```python
from build123d import *

# Parameters (mm, degrees)
CROQUIS1_W              = 65
CROQUIS1_H              = 65
CROQUIS1_R              = 5.1
CROQUIS1_R_2            = 6
CROQUIS1_R_3            = 4.6
SALIENTE_EXTRUIR1_DEPTH = 5
REDONDEO2_R             = 3
CROQUIS2_R              = 4.6
SALIENTE_EXTRUIR2_DEPTH = 1
CROQUIS3_R              = 2.5
CORTAR_EXTRUIR1_DEPTH   = 1
CROQUIS4_R              = 2.4
CORTAR_EXTRUIR2_DEPTH   = 10
CROQUIS5_R              = 2.4
CROQUIS5_R_2            = 1.25
SALIENTE_EXTRUIR3_DEPTH = 2.4
SALIENTE_EXTRUIR4_START = -2
CROQUIS6_R              = 5.1
SALIENTE_EXTRUIR4_DEPTH = 2


with BuildPart() as part:
    # Croquis1 → Saliente-Extruir1 (new body)
    with BuildSketch(Plane.XZ):
        with Locations((-15.241230111, -32.770729042)):
            Rectangle(CROQUIS1_W, CROQUIS1_H)
        with Locations((-35.389174066, -12.520729042)):
            Circle(CROQUIS1_R, mode=Mode.SUBTRACT)
        with Locations((4.310825934, -12.520729042)):
            Circle(CROQUIS1_R, mode=Mode.SUBTRACT)
        with Locations((-35.389174066, -52.520729042)):
            Circle(CROQUIS1_R, mode=Mode.SUBTRACT)
        with Locations((4.310825934, -52.520729042)):
            Circle(CROQUIS1_R, mode=Mode.SUBTRACT)
        with Locations((4.310825934, -32.520729042)):
            Circle(CROQUIS1_R_2, mode=Mode.SUBTRACT)
        with Locations((-35.389174066, -32.520729042)):
            Circle(CROQUIS1_R_3, mode=Mode.SUBTRACT)
        with BuildLine():
            Line((-32.439174066, -6.320729042), (-38.939173538, -6.320729042))
            ThreePointArc((-38.939173538, -6.320729042), (-40.439173538, -4.820729042), (-38.939173538, -3.320729042))
            Line((-38.939173538, -3.320729042), (-32.439174066, -3.320729042))
            ThreePointArc((-32.439174066, -3.320729042), (-30.939174066, -4.820729042), (-32.439174066, -6.320729042))
        make_face(mode=Mode.SUBTRACT)
        with BuildLine():
            Line((7.860825934, -6.320729042), (1.360825562, -6.320729042))
            ThreePointArc((1.360825562, -6.320729042), (-0.139174438, -4.820729042), (1.360825562, -3.320729042))
            Line((1.360825562, -3.320729042), (7.860825934, -3.320729042))
            ThreePointArc((7.860825934, -3.320729042), (9.360825934, -4.820729042), (7.860825934, -6.320729042))
        make_face(mode=Mode.SUBTRACT)
        with BuildLine():
            Line((-38.939173538, -58.720729042), (-32.439174066, -58.720729042))
            ThreePointArc((-32.439174066, -58.720729042), (-30.939174066, -60.220729042), (-32.439174066, -61.720729042))
            Line((-32.439174066, -61.720729042), (-38.939173538, -61.720729042))
            ThreePointArc((-38.939173538, -61.720729042), (-40.439173538, -60.220729042), (-38.939173538, -58.720729042))
        make_face(mode=Mode.SUBTRACT)
        with BuildLine():
            Line((7.860825934, -61.720729042), (1.360825562, -61.720729042))
            ThreePointArc((1.360825562, -61.720729042), (-0.139174438, -60.220729042), (1.360825562, -58.720729042))
            Line((1.360825562, -58.720729042), (7.860825934, -58.720729042))
            ThreePointArc((7.860825934, -58.720729042), (9.360825934, -60.220729042), (7.860825934, -61.720729042))
        make_face(mode=Mode.SUBTRACT)
    extrude(amount=SALIENTE_EXTRUIR1_DEPTH)

    # Redondeo2
    redondeo2_edges = [part.edges().sort_by_distance(p)[0] for p in [
        (-47.741230111, -2.5, -0.270729042),
        (17.258769889, -2.5, -0.270729042),
        (17.258769889, -2.5, -65.270729042),
        (-47.741230111, -2.5, -65.270729042),
    ]]
    fillet(redondeo2_edges, radius=REDONDEO2_R)

    # Croquis2 → Saliente-Extruir2 (add)
    with BuildSketch(Plane(origin=(0, 0, 0), x_dir=(1, 0, 0), z_dir=(0, 1, 0))):
        with Locations(Location((-35.389174066, 32.520729042, 0), (0, 0, 180))):
            Circle(CROQUIS2_R)
    extrude(amount=-SALIENTE_EXTRUIR2_DEPTH)

    # Croquis3 → Cortar-Extruir1 (cut)
    with BuildSketch(Plane.XZ.offset(1)):
        with Locations((-35.389174066, -32.520729042)):
            Circle(CROQUIS3_R)
    extrude(amount=-CORTAR_EXTRUIR1_DEPTH, mode=Mode.SUBTRACT)

    # Croquis4 → Cortar-Extruir2 (cut)
    with BuildSketch(Plane.XZ.offset(5)):
        with Locations((-35.241230111, -44.020729042)):
            Circle(CROQUIS4_R)
        with Locations((-35.241230111, -21.520729042)):
            Circle(CROQUIS4_R)
        with Locations((4.758769889, -21.520729042)):
            Circle(CROQUIS4_R)
        with Locations((4.758769889, -44.020729042)):
            Circle(CROQUIS4_R)
    extrude(amount=-CORTAR_EXTRUIR2_DEPTH, mode=Mode.SUBTRACT)

    # Croquis5 → Saliente-Extruir3 (add)
    # profile 1 of 4: a face of its own
    with BuildSketch(Plane.XZ.offset(5)):
        with Locations((-35.241230111, -44.020729042)):
            Circle(CROQUIS5_R)
        with Locations((-35.241230111, -44.020729042)):
            Circle(CROQUIS5_R_2, mode=Mode.SUBTRACT)
    # profile 2 of 4: a face of its own
    with BuildSketch(Plane.XZ.offset(5)):
        with Locations((-35.241230111, -21.520729042)):
            Circle(CROQUIS5_R)
        with Locations((-35.241230111, -21.520729042)):
            Circle(CROQUIS5_R_2, mode=Mode.SUBTRACT)
    # profile 3 of 4: a face of its own
    with BuildSketch(Plane.XZ.offset(5)):
        with Locations((4.758769889, -21.520729042)):
            Circle(CROQUIS5_R)
        with Locations((4.758769889, -21.520729042)):
            Circle(CROQUIS5_R_2, mode=Mode.SUBTRACT)
    # profile 4 of 4: a face of its own
    with BuildSketch(Plane.XZ.offset(5)):
        with Locations((4.758769889, -44.020729042)):
            Circle(CROQUIS5_R)
        with Locations((4.758769889, -44.020729042)):
            Circle(CROQUIS5_R_2, mode=Mode.SUBTRACT)
    extrude(amount=-SALIENTE_EXTRUIR3_DEPTH)

    # Croquis6 → Saliente-Extruir4 (add)
    with BuildSketch(Plane.XZ.offset(5).offset(SALIENTE_EXTRUIR4_START)):
        with Locations((-35.389174066, -52.520729042)):
            Circle(CROQUIS6_R)
        with Locations((4.310825934, -52.520729042)):
            Circle(CROQUIS6_R)
        with Locations((4.310825934, -12.520729042)):
            Circle(CROQUIS6_R)
        with Locations((-35.389174066, -12.520729042)):
            Circle(CROQUIS6_R)
    extrude(amount=SALIENTE_EXTRUIR4_DEPTH)


solid = part.part
```
Geometry check sheet. Reference: the model listing, model coordinates, mm. A direction names the side the tool comes from. Coordinates: 2 decimals unless noted, no trailing zeros. Order: outer loops, then holes, each group sorted by start corner. A loop starts at its lowest first (then second) coordinate and runs counter-clockwise, first axis right, second up. Notation, with made-up numbers: (65.5, 80) - (82.5, 80) arc R17 cw to (82.5, 90) - close; hole circle Ø7 at (12, 55). An arc over 180 degrees is marked (long way). Answer as a JSON object with one key per item and string values. Group by question number.
Item 1: Sectioned sample at C-C, the plane z = -49. Record the cut outline in (x, y), and give its area (3 significant figures).
Item 2: Sectioned sample at B-B, the plane z = -55.5. Record the cut outline in (x, y), and give its area (3 significant figures).
Item 3: Tool access check on faces 4 (the face through (3.2, -1.5, -57.5)), 5 (the face through (5, -2, -6.321)). Record the directions out of +Z, -Z, +X, -X, +Y, -Y that give a thin tool (end or side, any length) a straight path to the whole face; none if there is none.
Item 4: Depth check by flat-ended pin: pin 1 Ø5 at (x, z) = (3.5, -51) entering from +Y; pin 2 Ø1.4 at (x, z) = (-35.5, -21) entering from +Y; pin 3 Ø3 at (x, z) = (-33.5, -34.5) entering from -Y; pin 4 Ø3 at (x, z) = (-35.39, -32.52) entering from +Y. Enter the tip coordinate at first touch or a pass-through.
Item 5: Draft check along X on faces 1 (the face through (-36, -2, -6.321)), 2 (the face through (17.259, -2, -33)), 3 (the face through (4.6, -3.82, -42.78)). Enter one of: +X half, -X half, draft (parallel to the pull), parting line (faces both ways), or undercut.
Item 6: Scan lines: probe 1 along X at (y, z) = (-3.95, -4.5); probe 2 along X at (y, z) = (-1.6, -32.5); probe 3 along Z at (x, y) = (-40, -0.15). Record each from-to range of solid material in increasing order.
Item 7: Sectioned sample at A-A, the plane y = -1.75. Give the number of separate pieces and of enclosed holes in the cut face, and give its area (3 significant figures).
Resolved:
{
 "1": {"outline": "(-47.74, -5) - (17.26, -5) - (17.26, 0) - (8, 0) - (8, -3) - (0.62, -3) - (0.62, 0) - (-31.7, 0) - (-31.7, -3) - (-39.08, -3) - (-39.08, 0) - (-47.74, 0) - close", "area": "281 mm^2"},
 "2": {"outline": "(-47.74, -5) - (17.26, -5) - (17.26, 0) - (8.45, 0) - (8.45, -3) - (0.17, -3) - (0.17, 0) - (-31.25, 0) - (-31.25, -3) - (-39.53, -3) - (-39.53, 0) - (-47.74, 0) - close", "area": "275 mm^2"},
 "3": {"face 4": "+Y", "face 5": "+Y, -Y"},
 "4": {"pin 1": "y = -3", "pin 2": "y = -2.6", "pin 3": "y = -1", "pin 4": "through"},
 "5": {"face 1": "undercut", "face 2": "+X half", "face 3": "undercut"},
 "6": {"probe 1": "-47.74 to -40.4, -30.97 to -0.1, 9.33 to 17.26", "probe 2": "-47.74 to -39.99, -30.79 to -1.69, 10.31 to 17.26", "probe 3": "-65.27 to -61.28, -59.16 to -54.7, -50.34 to -14.7, -10.34 to -5.88, -3.76 to -0.27"},
 "7": {"separate pieces": "1", "enclosed holes": "14", "area": "3,530 mm^2"}
}
